```python
from build123d import *

# Parameters (mm, degrees)
SKETCH1_W           = 42.3
SKETCH1_H           = 42.3
BOSS_EXTRUDE1_DEPTH = 34
CHAMFER1_SIZE       = 5
SKETCH2_R           = 18
BOSS_EXTRUDE2_DEPTH = 27.3
SKETCH3_R           = 11
BOSS_EXTRUDE3_DEPTH = 2
SKETCH4_R           = 3
BOSS_EXTRUDE4_DEPTH = 16
CHAMFER2_SIZE       = 1
CHAMFER3_SIZE       = 0.5
SKETCH5_R           = 1.5
CUT_EXTRUDE1_DEPTH  = 5


with BuildPart() as part:
    # Sketch1 → Boss-Extrude1 (new body)
    with BuildSketch(Plane.XY):
        Rectangle(SKETCH1_W, SKETCH1_H)
    extrude(amount=BOSS_EXTRUDE1_DEPTH)

    # Chamfer1
    chamfer1_edges = [part.edges().sort_by_distance(p)[0] for p in [
        (21.15, -21.15, 17),
        (-21.15, -21.15, 17),
        (-21.15, 21.15, 17),
        (21.15, 21.15, 17),
    ]]
    chamfer(chamfer1_edges, length=CHAMFER1_SIZE)

    # Sketch2 → Boss-Extrude2 (add)
    with BuildSketch(Plane.XY.offset(34)):
        Circle(SKETCH2_R)
    extrude(amount=BOSS_EXTRUDE2_DEPTH)

    # Sketch3 → Boss-Extrude3 (add)
    with BuildSketch(Plane.XY.offset(61.3)):
        Circle(SKETCH3_R)
    extrude(amount=BOSS_EXTRUDE3_DEPTH)

    # Sketch4 → Boss-Extrude4 (add)
    with BuildSketch(Plane.XY.offset(63.3)):
        Circle(SKETCH4_R)
    extrude(amount=BOSS_EXTRUDE4_DEPTH)

    # Chamfer2
    chamfer2_edges = [part.edges().sort_by_distance(p)[0] for p in [
        (0, -21.15, 0),
        (0, -21.15, 34),
        (21.15, 0, 0),
        (-21.15, 0, 0),
        (0, 21.15, 0),
        (18.65, 18.65, 0),
        (18.65, -18.65, 0),
        (-18.65, 18.65, 0),
        (-18.65, -18.65, 0),
        (-21.15, 0, 34),
        (21.15, 0, 34),
        (0, 21.15, 34),
        (18.65, 18.65, 34),
        (18.65, -18.65, 34),
        (-18.65, 18.65, 34),
        (-18.65, -18.65, 34),
        (-18, 0, 34),
        (-18, 0, 61.3),
        (-11, 0, 63.3),
    ]]
    chamfer(chamfer2_edges, length=CHAMFER2_SIZE)

    # Chamfer3
    chamfer3_edges = [part.edges().sort_by_distance(p)[0] for p in [
        (-3, 0, 79.3),
    ]]
    chamfer(chamfer3_edges, length=CHAMFER3_SIZE)

    # Sketch5 → Cut-Extrude1 (cut)
    with BuildSketch(Plane.XY.offset(61.3)):
        with Locations((9.899494937, 9.899494937)):
            Circle(SKETCH5_R)
        with Locations((9.899494937, -9.899494937)):
            Circle(SKETCH5_R)
        with Locations((-9.899494937, -9.899494937)):
            Circle(SKETCH5_R)
        with Locations((-9.899494937, 9.899494937)):
            Circle(SKETCH5_R)
    extrude(amount=-CUT_EXTRUDE1_DEPTH, mode=Mode.SUBTRACT)


solid = part.part
```
Geometry: final body of the model. Coordinates: model frame, mm. A direction names the side the tool comes from. Coordinates: 2 decimals unless noted, no trailing zeros. Order: outer loops, then holes, each group sorted by start corner. A loop starts at its lowest first (then second) coordinate and runs counter-clockwise, first axis right, second up. Notation, with made-up numbers: (-34, -15.5) -> (-25, -15.5) arc R5 cw to (-25, -10.5) -> close; hole circle Ø9 at (5.5, 38.25). An arc over 180 degrees is marked (long way). Write item = value, one per line.
(1) Line query: line 1 (Z direction, x = 2.5, y = 13.5); line 2 (Z direction, x = -15, y = -13); line 3 (X direction, y = -10.5, z = 60). Output: solid intervals per line, ascending.
Solved:
line_1 = 0 to 61.3
line_2 = 0 to 34
line_3 = -14.62 to -11.27, -8.52 to 8.52, 11.27 to 14.62
(2) Cut plane C-C on z = 19. Return loops of the section in (x, y).
Solved:
outline = (-21.15, -16.15) -> (-16.15, -21.15) -> (16.15, -21.15) -> (21.15, -16.15) -> (21.15, 16.15) -> (16.15, 21.15) -> (-16.15, 21.15) -> (-21.15, 16.15) -> close
(3) Access query for faces 4 (the flat face through (0, 0, 79.3)), 5 (the cylindrical face through (-9.093, -8.635, 58.835)). Directions: +Z, -Z, +X, -X, +Y, -Y. A direction counts if a zero-diameter tool reaches every point of the face in a straight line with its end or side. Return the directions, or none.
Solved:
face_4 = +Z, +X, -X, +Y, -Y
face_5 = +Z
(4) Pin query (flat end, axial travel): pin 1 Ø3.5 at (x, y) = (-9.9, 9.9) entering from +Z; pin 2 Ø8 at (y, z) = (10, 68) entering from +X; pin 3 Ø6 at (x, z) = (1.5, 48.5) entering from -Y; pin 4 Ø10 at (x, z) = (-14.5, 38.5) entering from -Y. Return the tip coordinate at first contact, or that it passes through.
Solved:
pin_1 = 61.3
pin_2 = through
pin_3 = -18
pin_4 = -20.65
(5) Pull-direction query (X, two-part tool) for faces 1 (the flat face through (10, -10, 56.3)), 2 (the cylindrical face through (-3, 0, 71)), 3 (the flat face through (4, -11, 61.3)); classes: pulls with the +X half, pulls with the -X half, needs draft (parallel to the pull), parting line crosses it, or undercut.
Solved:
face_1 = undercut
face_2 = parting line crosses it
face_3 = needs draft
(6) Cut plane A-A on x = 0. Return loops of the section in (y, z), plus the area to 3 significant figures.
Solved:
outline = (-21.15, 1) -> (-20.15, 0) -> (20.15, 0) -> (21.15, 1) -> (21.15, 33) -> (20.15, 34) -> (19, 34) -> (18, 35) -> (18, 60.3) -> (17, 61.3) -> (11, 61.3) -> (11, 62.3) -> (10, 63.3) -> (3, 63.3) -> (3, 78.8) -> (2.5, 79.3) -> (-2.5, 79.3) -> (-3, 78.8) -> (-3, 63.3) -> (-10, 63.3) -> (-11, 62.3) -> (-11, 61.3) -> (-17, 61.3) -> (-18, 60.3) -> (-18, 35) -> (-19, 34) -> (-20.15, 34) -> (-21.15, 33) -> close
area = 2,560 mm²
